Could you check a few things on this drawing? It's one solid part, dimensions in mm from its lowest x, y, z. A direction names the side the tool comes from. Give positions to 0.01 mm unless a question says otherwise; leave off trailing zeros. Write each loop counter-clockwise with the first axis right and the second up, starting at its lowest first coordinate (ties: lowest second). Pieces come first, ordered by that corner, then holes. Notation, with made-up numbers: (25.5, 7) -> (32.5, 7) arc R32 cw to (32.5, 40) -> close; hole circle Ø5 at (-0.5, -24). An arc over 180 degrees is marked (long way). Use CSV: the item, a comma, the result in double quotes. Start each with the question number.
(1) Which directions (+Z, -Z, +X, -X, +Y, -Y) give clear straight access to the entire face, cutting with the end or side of a thin tool? Please do the marked faces 1, 2, 3 and 4.
(2) Suppose I cut it at A-A on x = 110.2. List the corners of the cut face in (y, z) for me, plus the area to 3 significant figures.
(3) Suppose I cut it at B-B on z = 6.5. List the corners of the cut face in (x, y) for me, plus the area to 4 significant figures.
(4) Suppose I cut it at C-C on y = 42.5. List the corners of the cut face in (x, z) for me.
(5) For pin 1 Ø3.5 at (x, y) = (11, 8) entering from -Z; pin 2 Ø6 at (x, z) = (18, 14) entering from +Y; pin 3 Ø4 at (x, z) = (5, 10) entering from -Y, each with a flat end and sliding along its axis, tell me the tip position at first contact or that it passes through.
(6) I need wall thicknesses on L1, parallel to X at y = 9, z = 32.5; L2, parallel to Y at x = 102, z = 32.5; L3, parallel to X at y = 43, z = 17. Which ranges of each line are inside material? Lowest first, please. Write a range as [from, to].
(7) Suppose I cut it at D-D on x = 72.5. List the corners of the cut face in (y, z) for me.
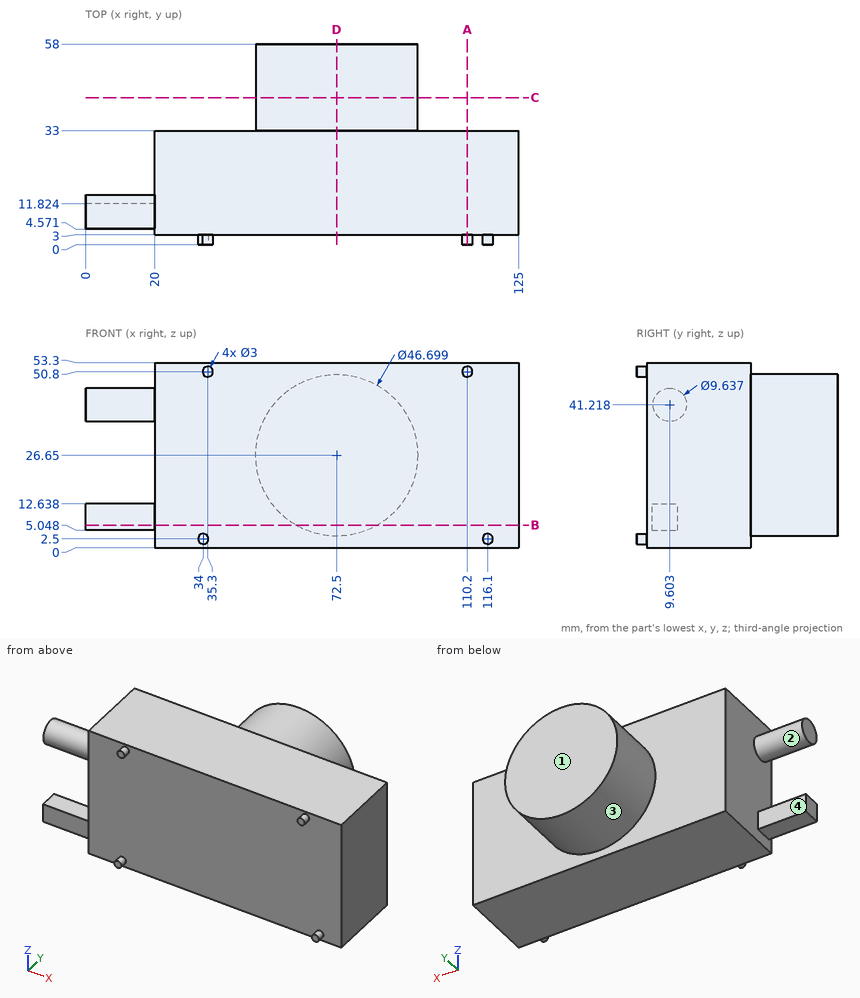
Geometry says:
1,face 1,"+Z, -Z, +X, -X, +Y"
1,face 2,"-X"
1,face 3,"+Y"
1,face 4,"-Z, -X, +Y"
2,outline,"(0, 49.3) -> (3, 49.3) -> (3, 0) -> (33, 0) -> (33, 53.3) -> (3, 53.3) -> (3, 52.3) -> (0, 52.3) -> close"
2,area,"1,610 mm²"
3,outline,"(0, 4.57) -> (20, 4.57) -> (20, 3) -> (125, 3) -> (125, 33) -> (84.3, 33) -> (84.3, 58) -> (60.7, 58) -> (60.7, 33) -> (20, 33) -> (20, 11.82) -> (0, 11.82) -> close"
3,area,"3,885 mm²"
4,outline,"circle Ø46.7 at (72.5, 26.65)"
5,pin 1,"z = 5.05"
5,pin 2,"y = 33"
5,pin 3,"y = 4.57"
6,L1,"[20, 125]"
6,L2,"[3, 33]"
6,L3,"[51.24, 93.76]"
7,outline,"(3, 0) -> (33, 0) -> (33, 3.3) -> (58, 3.3) -> (58, 50) -> (33, 50) -> (33, 53.3) -> (3, 53.3) -> close"
